Could you check a few things on this model? Use its own coordinates, in mm. A direction names the side the tool comes from. Give positions to 0.01 mm unless a question says otherwise; leave off trailing zeros. Write each loop counter-clockwise with the first axis right and the second up, starting at its lowest first coordinate (ties: lowest second). Pieces come first, ordered by that corner, then holes. Notation, with made-up numbers: (-13, 17) - (33, 17) arc R25 cw to (33, 32) - close; hole circle Ø5 at (15, -13). An arc over 180 degrees is marked (long way). Answer in a Markdown table with one row per item.
from build123d import *

# Parameters (mm, degrees)
BOSS_EXTRUDE1_DEPTH = 30
SKETCH2_R           = 25
CUT_EXTRUDE1_DEPTH  = 30
SKETCH3_R           = 6.505
BOSS_EXTRUDE2_DEPTH = 40
CUT_EXTRUDE2_DEPTH  = 40


with BuildPart() as part:
    # Sketch1 → Boss-Extrude1 (new body)
    with BuildSketch(Plane(origin=(0, 0, 0), x_dir=(1, 0, 0), z_dir=(0, 1, 0))):
        with BuildLine():
            Line((-77.61802258, 0), (-33.820586084, 266.179413916))
            ThreePointArc((-33.820586084, 266.179413916), (0, 300), (33.820586084, 266.179413916))
            Line((33.820586084, 266.179413916), (72.176610565, 0))
            Line((72.176610565, 0), (33.820586084, -266.179413916))
            ThreePointArc((33.820586084, -266.179413916), (0, -300), (-33.820586084, -266.179413916))
            Line((-33.820586084, -266.179413916), (-77.61802258, 0))
        make_face()
    extrude(amount=BOSS_EXTRUDE1_DEPTH)

    # Sketch2 → Cut-Extrude1 (cut)
    with BuildSketch(Plane(origin=(0, 30, 0), x_dir=(1, 0, 0), z_dir=(0, 1, 0))):
        Circle(SKETCH2_R)
    extrude(amount=-CUT_EXTRUDE1_DEPTH, mode=Mode.SUBTRACT)

    # Sketch3 → Boss-Extrude2 (add)
    with BuildSketch(Plane(origin=(0, 30, 0), x_dir=(1, 0, 0), z_dir=(0, 1, 0))):
        with Locations((0, -280)):
            Circle(SKETCH3_R)
    boss_extrude2 = extrude(amount=BOSS_EXTRUDE2_DEPTH)

    # Mirror1: Boss-Extrude2 across plane
    add(boss_extrude2.mirror(Plane.XY))

    # Sketch4 → Cut-Extrude2 (cut)
    with BuildSketch(Plane(origin=(0, 30, 0), x_dir=(1, 0, 0), z_dir=(0, 1, 0))):
        with BuildLine():
            Line((-77.61802258, 0), (-33.820586084, -266.179413916))
            add(Edge.make_bspline(
                [(-33.820586084, 266.179413916), (-66.842002298, 0), (-33.820586084, -266.179413916)],
                knots=[0, 0, 0, 1, 1, 1], degree=2))
            add(Edge.make_bspline(
                [(-33.820586084, 266.179413916), (-77.61802258, 0)],
                knots=[0, 0, 1, 1], degree=1))
        make_face()
        with BuildLine():
            Line((72.176610565, 0), (33.820586084, 266.179413916))
            add(Edge.make_bspline(
                [(33.820586084, 266.179413916), (60.12786219, -0.030187119), (33.820586084, -266.179413916)],
                knots=[0, 0, 0, 1, 1, 1], degree=2))
            Line((33.820586084, -266.179413916), (72.176610565, 0))
        make_face()
    extrude(amount=-CUT_EXTRUDE2_DEPTH, mode=Mode.SUBTRACT)


solid = part.part
1) Imagine slicing it at C-C (z = -280). List the corners of the cut face in (x, y) for me (3 decimals).
Check values:
| item | result |
|---|---|
| outline | (-30.868, 0) - (30.868, 0) - (30.868, 30) - (6.505, 30) - (6.505, 70) - (-6.505, 70) - (-6.505, 30) - (-30.868, 30) - close |
2) Imagine slicing it at A-A (x = 0). List the corners of the cut face in (y, z) for me (3 decimals), then the cut area to 3 significant figures.
Check values:
| item | result |
|---|---|
| outline | (0, -300) - (30, -300) - (30, -286.505) - (70, -286.505) - (70, -273.495) - (30, -273.495) - (30, -25) - (0, -25) - close; (0, 25) - (30, 25) - (30, 273.495) - (70, 273.495) - (70, 286.505) - (30, 286.505) - (30, 300) - (0, 300) - close |
| area | 17,500 mm2 |
3) Will these pins go through, and if not, where does the flat tip stop? P1, Ø3, axis at x = -28.5, z = -98.5, coming from the -Y side; P2, Ø1.5, axis at x = -28.5, z = -198.5, coming from the +Y side; P3, Ø1.5, axis at x = 17.5, y = 10.5, coming from the +Z side; P4, Ø3, axis at x = 5.5, y = 14.5, coming from the -Z side.
Check values:
| item | result |
|---|---|
| P1 | stops at y = 0 |
| P2 | stops at y = 30 |
| P3 | stops at z = 295.56 |
| P4 | stops at z = -299.76 |
4) On a 3-axis mill with a long thin cutter (end or side, diameter ignored), from which of +Z, -Z, +X, -X, +Y, -Y can I reach the whole of each face in a straight line? I mean faces 4 (the face through (0, 70, -280)), 5 (the face through (-0.85, 49.72, -273.55)). Say none if no direction works.
Check values:
| item | result |
|---|---|
| face 4 | +Z, -Z, +X, -X, +Y |
| face 5 | +Y |
5) We'd pull the mould along Z, two halves only. Please class faces 1 (the face through (-33, 0, -4)), 2 (the face through (-0.85, 49.72, 273.55)), 3 (the face through (-0.74, 14.79, -299.99)): +Z half, -Z half, draft (parallel to the pull), parting line (faces both ways), or undercut.
Check values:
| item | result |
|---|---|
| face 1 | draft |
| face 2 | undercut |
| face 3 | -Z half |
6) If I drill on line 1 (X direction, y = 6, z = 0); line 2 (Z direction, x = 0, y = 22), over which ranges is the centre line in solid material (lowest first)?
Check values:
| item | result |
|---|---|
| line 1 | x = -50.33 to -25, 25 to 46.97 |
| line 2 | z = -300 to -25, 25 to 300 |
7) Imagine slicing it at B-B (y = 48). List the corners of the cut face in (x, z) for me (3 decimals), then the cut area to 3 significant figures.
Check values:
| item | result |
|---|---|
| outline | circle Ø13.01 at (0, -280); circle Ø13.01 at (0, 280) |
| area | 266 mm2 |
